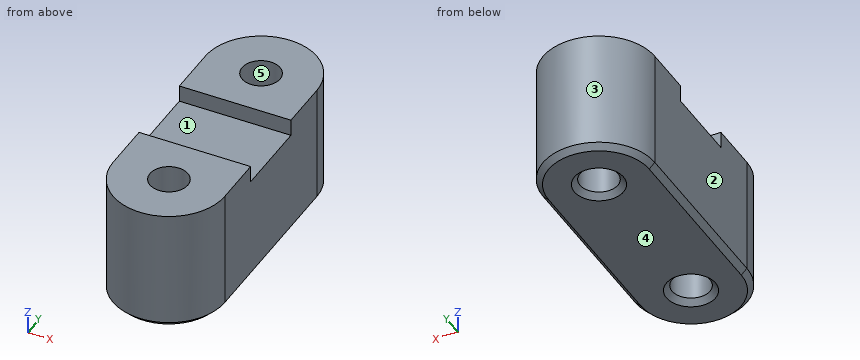
from build123d import *

# Parameters (mm, degrees)
SKETCH1_R           = 1.7
BOSS_EXTRUDE1_DEPTH = 11
SKETCH2_W           = 10
SKETCH2_H           = 7
CUT_EXTRUDE1_DEPTH  = 1.5
CHAMFER1_SIZE       = 0.5


with BuildPart() as part:
    # Sketch1 → Boss-Extrude1 (new body)
    with BuildSketch(Plane.XY):
        with BuildLine():
            Line((-5, -8), (-5, 8))
            ThreePointArc((-5, 8), (0, 13), (5, 8))
            Line((5, 8), (5, -8))
            ThreePointArc((5, -8), (0, -13), (-5, -8))
        make_face()
        with Locations((0, 8)):
            Circle(SKETCH1_R, mode=Mode.SUBTRACT)
        with Locations((0, -8)):
            Circle(SKETCH1_R, mode=Mode.SUBTRACT)
    extrude(amount=BOSS_EXTRUDE1_DEPTH)

    # Sketch2 → Cut-Extrude1 (cut)
    with BuildSketch(Plane.XY.offset(11)):
        Rectangle(SKETCH2_W, SKETCH2_H)
    extrude(amount=-CUT_EXTRUDE1_DEPTH, mode=Mode.SUBTRACT)

    # Chamfer1
    chamfer1_edges = [part.edges().sort_by_distance(p)[0] for p in [
        (-1.7, 8, 0),
        (-1.7, -8, 0),
        (-5, 0, 0),
        (0, 13, 0),
        (5, 0, 0),
        (0, -13, 0),
    ]]
    chamfer(chamfer1_edges, length=CHAMFER1_SIZE)


solid = part.part
The listing builds one solid part. Answer for the finished solid, in the listing's coordinates (mm). Face numbers are marked on the shaded views. A direction names the side the tool comes from. Coordinates: 2 decimals unless noted, no trailing zeros. Order: outer loops, then holes, each group sorted by start corner. A loop starts at its lowest first (then second) coordinate and runs counter-clockwise, first axis right, second up.
Q1. A cutting plane is placed at A-A, the plane x = 0. Write down the section's boundary in (y, z), and give its area (3 significant figures).
Q2. Given P1, Ø3, axis at x = -2.5, z = 8, coming from the -Y side; P2, Ø0.8, axis at x = -2, z = 10, coming from the -Y side; P3, Ø6, axis at x = 3.5, z = 5, coming from the +Y side, each flat-ended and moving along its own axis, determine where each tip first touches the part or whether it passes through.
Q3. Which of the six approach directions +Z, -Z, +X, -X, +Y, -Y give full straight-line access (tool end or side, diameter ignored) to the marked faces 1 and 2?
Q4. Consider line 1 (Y direction, x = 0, z = 4.5); line 2 (Y direction, x = 0.75, z = 9.25); line 3 (X direction, y = -7.75, z = 5.25). Determine where each line is inside the solid, lowest interval first.
Q5. For a pull along X with two mould halves and no side action, classify the marked faces 3, 4 and 5 as pulls with the +X half, pulls with the -X half, needs draft (parallel to the pull), parting line crosses it, or undercut.
Q6. A cutting plane is placed at C-C, the plane y = -3. Write down the section's boundary in (x, z), and give its area (4 significant figures).
Q7. A cutting plane is placed at B-B, the plane z = 7.5. Write down the section's boundary in (x, y).
Answers follow:
1. outline: (-13, 0.5) - (-12.5, 0) - (-10.2, 0) - (-9.7, 0.5) - (-9.7, 11) - (-13, 11) - close; (-6.3, 0.5) - (-5.8, 0) - (5.8, 0) - (6.3, 0.5) - (6.3, 11) - (3.5, 11) - (3.5, 9.5) - (-3.5, 9.5) - (-3.5, 11) - (-6.3, 11) - close; (9.7, 0.5) - (10.2, 0) - (12.5, 0) - (13, 0.5) - (13, 11) - (9.7, 11) - close
1. area: 200 mm2
2. P1: stops at y = -12.9
2. P2: stops at y = -12.74
2. P3: stops at y = 12.97
3. face 1: +Z, +X, -X
3. face 2: +Z, -Z, -X, +Y, -Y
4. line 1: y = -13 to -9.7, -6.3 to 6.3, 9.7 to 13
4. line 2: y = -12.94 to -9.53, -6.47 to 6.47, 9.53 to 12.94
4. line 3: x = -5 to -1.68, 1.68 to 5
5. face 3: parting line crosses it
5. face 4: needs draft
5. face 5: undercut
6. outline: (-5, 0.5) - (-4.5, 0) - (4.5, 0) - (5, 0.5) - (5, 9.5) - (-5, 9.5) - close
6. area: 94.75 mm2
7. outline: (-5, -8) arc R5 ccw to (5, -8) - (5, 8) arc R5 ccw to (-5, 8) - close; hole circle Ø3.4 at (0, -8); hole circle Ø3.4 at (0, 8)
